```python
from build123d import *

# Parameters (mm, degrees)
SKETCH1_W                                 = 66.38
SKETCH1_H                                 = 120
BOSS_EXTRUDE1_DEPTH                       = 6.35
SKETCH2_W                                 = 40.98
SKETCH2_H                                 = 7.7
CUT_EXTRUDE1_DEPTH                        = 121
F_3_32_0_09375_DIAMETER_HOLE1_D           = 2.38125
F_3_32_0_09375_DIAMETER_HOLE1_DEPTH       = 19.05
F_3_32_0_09375_DIAMETER_HOLE1_CSINK_D     = 3.175
F_3_32_0_09375_DIAMETER_HOLE1_CSINK_ANGLE = 90
F_3_32_0_09375_DIAMETER_HOLE1_TIP         = 0.715399675
CUT_EXTRUDE2_DEPTH                        = 1
CUT_EXTRUDE2_DEPTH_BACK                   = 121
F_5_16_18_TAPPED_HOLE1_D                  = 6.5278
F_5_16_18_TAPPED_HOLE1_DEPTH              = 32.45
F_5_16_18_TAPPED_HOLE1_CSINK_D            = 9.2075
F_5_16_18_TAPPED_HOLE1_CSINK_ANGLE        = 90
F_5_16_18_TAPPED_HOLE1_TIP                = 1.961148974
CHAMFER1_SIZE                             = 3.175
SKETCH6_W                                 = 15.1
SKETCH6_H                                 = 7.75
CUT_EXTRUDE3_DEPTH                        = 6
FILLET1_R                                 = 1
SKETCH18_W                                = 14.39
SKETCH18_H                                = 120
CUT_EXTRUDE10_DEPTH                       = 13.7000001
SKETCH19_W                                = 5
SKETCH19_H                                = 12.7
BOSS_EXTRUDE3_DEPTH                       = 7.7
SKETCH20_W                                = 12.7
SKETCH20_H                                = 3
BOSS_EXTRUDE4_DEPTH                       = 1.1
CHAMFER3_SIZE                             = 1
CHAMFER4_SIZE                             = 2
SKETCH21_W                                = 12.7
SKETCH21_H                                = 100.95
CUT_EXTRUDE11_DEPTH                       = 7.7
SKETCH22_W                                = 24.87086649
SKETCH22_H                                = 0.4
CUT_EXTRUDE12_DEPTH                       = 121.0000001
SKETCH23_W                                = 40.98
SKETCH23_H                                = 0.68791644
CUT_EXTRUDE13_DEPTH                       = 121
CHAMFER5_SIZE                             = 2


with BuildPart() as part:
    # Sketch1 → Boss-Extrude1 (new body, symmetric)
    with BuildSketch(Plane(origin=(0, 0, 0), x_dir=(1, 0, 0), z_dir=(0, 1, 0))):
        with Locations((0, 60)):
            Rectangle(SKETCH1_W, SKETCH1_H)
    extrude(amount=BOSS_EXTRUDE1_DEPTH, both=True)

    # Sketch2 → Cut-Extrude1 (cut, through all)
    with BuildSketch(Plane.XY):
        with Locations((0, 2.5)):
            Rectangle(SKETCH2_W, SKETCH2_H)
    extrude(amount=-CUT_EXTRUDE1_DEPTH, mode=Mode.SUBTRACT)

    # 3_32 _0.09375_ Diameter Hole1
    with Locations(Plane.XY):
        with Locations((0, -3.35)):
            CounterSinkHole(F_3_32_0_09375_DIAMETER_HOLE1_D / 2, F_3_32_0_09375_DIAMETER_HOLE1_CSINK_D / 2, depth=F_3_32_0_09375_DIAMETER_HOLE1_DEPTH, counter_sink_angle=F_3_32_0_09375_DIAMETER_HOLE1_CSINK_ANGLE)
            with Locations((0, 0, -(F_3_32_0_09375_DIAMETER_HOLE1_DEPTH + F_3_32_0_09375_DIAMETER_HOLE1_TIP / 2))):  # 118° drill point
                Cone(0, F_3_32_0_09375_DIAMETER_HOLE1_D / 2, F_3_32_0_09375_DIAMETER_HOLE1_TIP, mode=Mode.SUBTRACT)

    # Sketch3 → Cut-Extrude2 (cut, two sides)
    with BuildSketch(Plane.XY) as cut_extrude2_sk:
        with BuildLine():
            Line((-140.137251951, -19.091259006), (-20.49, -6.35))
            ThreePointArc((-20.49, -6.35), (0, -5.26208356), (20.49, -6.35))
            Line((20.49, -6.35), (140.137251951, -19.091259006))
            Line((140.137251951, -19.091259006), (140.137251951, -259.738757065))
            Line((140.137251951, -259.738757065), (-140.137251951, -259.738757065))
            Line((-140.137251951, -259.738757065), (-140.137251951, -19.091259006))
        make_face()
    extrude(amount=CUT_EXTRUDE2_DEPTH, mode=Mode.SUBTRACT)
    extrude(cut_extrude2_sk.sketch, amount=-CUT_EXTRUDE2_DEPTH_BACK, mode=Mode.SUBTRACT)

    # 5_16-18 Tapped Hole1
    with Locations(Plane.XY):
        with Locations((-26.84, 0)):
            CounterSinkHole(F_5_16_18_TAPPED_HOLE1_D / 2, F_5_16_18_TAPPED_HOLE1_CSINK_D / 2, depth=F_5_16_18_TAPPED_HOLE1_DEPTH, counter_sink_angle=F_5_16_18_TAPPED_HOLE1_CSINK_ANGLE)
            with Locations((0, 0, -(F_5_16_18_TAPPED_HOLE1_DEPTH + F_5_16_18_TAPPED_HOLE1_TIP / 2))):  # 118° drill point
                Cone(0, F_5_16_18_TAPPED_HOLE1_D / 2, F_5_16_18_TAPPED_HOLE1_TIP, mode=Mode.SUBTRACT)

    # Chamfer1
    chamfer1_edges = [part.edges().sort_by_distance(p)[0] for p in [
        (-20.49, 6.35, -60),
    ]]
    chamfer(chamfer1_edges, length=CHAMFER1_SIZE)

    # Sketch6 → Cut-Extrude3 (cut, through all)
    with BuildSketch(Plane(origin=(0, -1.35, 0), x_dir=(1, 0, 0), z_dir=(0, 1, 0))):
        with Locations((3.55, 107.9216)):
            Rectangle(SKETCH6_W, SKETCH6_H)
        with Locations((-2.75, 47.6216)):
            Rectangle(SKETCH6_W, SKETCH6_H)
    extrude(amount=-CUT_EXTRUDE3_DEPTH, mode=Mode.SUBTRACT)

    # Fillet1
    fillet1_edges = [part.edges().sort_by_distance(p)[0] for p in [
        (11.1, -3.465359, -111.7966),
        (11.1, -3.465359, -104.0466),
        (-4, -3.326715824, -104.0466),
        (-4, -3.326715824, -111.7966),
        (4.8, -3.335813803, -51.4966),
        (4.8, -3.335813803, -43.7466),
        (-10.3, -3.443206194, -43.7466),
        (-10.3, -3.443206194, -51.4966),
    ]]
    fillet(fillet1_edges, radius=FILLET1_R)

    # Sketch18 → Cut-Extrude10 (cut, through all)
    with BuildSketch(Plane(origin=(0, 6.35, 0), x_dir=(1, 0, 0), z_dir=(0, 1, 0))):
        with Locations((25.995, 60)):
            Rectangle(SKETCH18_W, SKETCH18_H)
    extrude(amount=-CUT_EXTRUDE10_DEPTH, mode=Mode.SUBTRACT)

    # Sketch19 → Boss-Extrude3 (add)
    with BuildSketch(Plane(origin=(0, -1.35, 0), x_dir=(1, 0, 0), z_dir=(0, 1, 0))):
        with Locations((16.3, 19.05)):
            Rectangle(SKETCH19_W, SKETCH19_H)
        with Locations((16.3, 82.55)):
            Rectangle(SKETCH19_W, SKETCH19_H)
    extrude(amount=BOSS_EXTRUDE3_DEPTH)

    # Sketch20 → Boss-Extrude4 (add)
    with BuildSketch(Plane(origin=(18.8, 0, 0), x_dir=(0, 0, -1), z_dir=(1, 0, 0))):
        with Locations((19.05, 4.85)):
            Rectangle(SKETCH20_W, SKETCH20_H)
        with Locations((82.55, 4.85)):
            Rectangle(SKETCH20_W, SKETCH20_H)
    extrude(amount=BOSS_EXTRUDE4_DEPTH)

    # Chamfer3
    chamfer3_edges = [part.edges().sort_by_distance(p)[0] for p in [
        (19.9, 3.35, -82.55),
        (19.9, 3.35, -19.05),
    ]]
    chamfer(chamfer3_edges, length=CHAMFER3_SIZE)

    # Chamfer4
    chamfer4_edges = [part.edges().sort_by_distance(p)[0] for p in [
        (13.8, 6.35, -19.05),
        (13.8, 6.35, -82.55),
    ]]
    chamfer(chamfer4_edges, length=CHAMFER4_SIZE)

    # Sketch21 → Cut-Extrude11 (cut)
    with BuildSketch(Plane(origin=(0, 6.35, 0), x_dir=(1, 0, 0), z_dir=(0, 1, 0))):
        with Locations((-26.84, 69.525)):
            Rectangle(SKETCH21_W, SKETCH21_H)
    extrude(amount=-CUT_EXTRUDE11_DEPTH, mode=Mode.SUBTRACT)

    # Sketch22 → Cut-Extrude12 (cut, through all)
    with BuildSketch(Plane.XY):
        with Locations((0, -5.46208356)):
            Rectangle(SKETCH22_W, SKETCH22_H)
    extrude(amount=-CUT_EXTRUDE12_DEPTH, mode=Mode.SUBTRACT)

    # Sketch23 → Cut-Extrude13 (cut, through all)
    with BuildSketch(Plane.XY):
        with Locations((0, -6.00604178)):
            Rectangle(SKETCH23_W, SKETCH23_H)
    extrude(amount=-CUT_EXTRUDE13_DEPTH, mode=Mode.SUBTRACT)

    # Chamfer5
    chamfer5_edges = [part.edges().sort_by_distance(p)[0] for p in [
        (-2.75, -1.35, -51.4966),
        (4.8, -1.35, -47.6216),
        (-2.75, -1.35, -43.7466),
        (-10.3, -1.35, -47.6216),
        (-3.707106781, -1.35, -104.339493219),
        (10.807106781, -1.35, -104.339493219),
        (10.807106781, -1.35, -111.503706781),
        (4.507106781, -1.35, -51.203706781),
        (4.507106781, -1.35, -44.039493219),
        (-10.007106781, -1.35, -44.039493219),
        (-10.007106781, -1.35, -51.203706781),
        (-3.707106781, -1.35, -111.503706781),
        (3.55, -1.35, -104.0466),
        (-4, -1.35, -107.9216),
        (11.1, -1.35, -107.9216),
        (3.55, -1.35, -111.7966),
    ]]
    chamfer(chamfer5_edges, length=CHAMFER5_SIZE)


solid = part.part
```
Geometry check sheet. Reference: the model listing, model coordinates, mm. A direction names the side the tool comes from. Coordinates: 2 decimals unless noted, no trailing zeros. Loops run counter-clockwise (first coordinate to the right, second up) from the corner with the lowest first, then second, coordinate; pieces in that order, holes last. Notation, with made-up numbers: (82.5, 34.25) - (111.5, 34.25) arc R33 cw to (111.5, 64.25) - close; hole circle Ø5 at (46, -17). An arc over 180 degrees is marked (long way). One line per item, written item: value. Start each with the question number.
(1) Cross-section at A-A on y = 0. Enter the section's corners in (x, z).
(2) Cross-section at C-C on z = -87. Enter the section's corners in (x, y), plus the area to 3 significant figures.
(3) Cross-section at B-B on z = -15. Enter the section's corners in (x, y) (3 decimals).
(4) Material ranges on line 1 (X direction, y = 0, z = -15.5); line 2 (Z direction, x = 17, y = 3.25); line 3 (X direction, y = -3.35, z = -15), recorded low to high. Write a range as [from, to].
(5) Mould release check, pull along Z, two halves, no side actions. Record for faces 6 (the flat face through (17, 2, -25.4)), 7 (the flat face through (-2.842, -2.364, -52.483)), 8 (the flat face through (-33.19, -3, -46)), 9 (the flat face through (-8, -3, -120)): released by +Z, released by -Z, zero draft, split by the parting line, or undercut.
(6) Tool access check on faces 1 (the flat face through (18, 6.35, -83)), 2 (the flat face through (16, -5.662, -59)), 3 (the flat face through (-2.658, -2.364, -42.761)), 4 (the flat face through (14.79, 5.34, -18.96)), 5 (the flat face through (19.9, 5, -82)). Record the directions out of +Z, -Z, +X, -X, +Y, -Y that give a thin tool (end or side, any length) a straight path to the whole face; none if there is none.
(7) Depth check by flat-ended pin: P1, Ø2, axis at y = 0, z = -12.5, coming from the +X side; P2, Ø2, axis at x = -0.5, y = -4.5, coming from the +Z side; P3, Ø1.8, axis at x = 18, y = 0.5, coming from the +Z side; P4, Ø1, axis at x = -11, z = -70.5, coming from the -Y side. Enter the tip coordinate at first touch or a pass-through.
Results below:
1. outline: (-33.19, -19.05) - (-30.1, -19.05) - (-30.1, -1.34) - (-31.44, 0) - (-33.19, 0) - close; (-23.58, -19.05) - (-20.49, -19.05) - (-20.49, 0) - (-22.24, 0) - (-23.58, -1.34) - close; (13.8, -88.9) - (18.8, -88.9) - (18.8, -76.2) - (13.8, -76.2) - close; (13.8, -25.4) - (18.8, -25.4) - (18.8, -12.7) - (13.8, -12.7) - close
2. outline: (-33.19, -6.35) - (-20.49, -6.35) - (-20.49, -5.66) - (-12.44, -5.66) - (-12.44, -5.26) - (12.44, -5.26) - (12.44, -5.66) - (18.8, -5.66) - (18.8, 3.35) - (18.9, 3.35) - (19.9, 4.35) - (19.9, 6.35) - (15.8, 6.35) - (13.8, 4.35) - (13.8, -1.35) - (-33.19, -1.35) - close
2. area: 262 mm2
3. outline: (-33.19, -6.35) - (-20.49, -6.35) - (-20.49, -5.662) - (-12.435, -5.662) - (-12.435, -5.262) - (12.435, -5.262) - (12.435, -5.662) - (18.8, -5.662) - (18.8, 3.35) - (18.9, 3.35) - (19.9, 4.35) - (19.9, 6.35) - (15.8, 6.35) - (13.8, 4.35) - (13.8, -1.35) - (-20.49, -1.35) - (-20.49, 3.175) - (-23.665, 6.35) - (-33.19, 6.35) - close; hole circle Ø6.528 at (-26.84, 0); hole circle Ø2.381 at (0, -3.35)
4. line 1: x = [-33.19, -30.1], [-23.58, -20.49], [13.8, 18.8]
4. line 2: z = [-88.9, -76.2], [-25.4, -12.7]
4. line 3: x = [-33.19, -1.19], [1.19, 18.8]
5. face 6: undercut
5. face 7: undercut
5. face 8: zero draft
5. face 9: released by -Z
6. face 1: +Z, -Z, +X, -X, +Y
6. face 2: +Z, -Z, +X, -Y
6. face 3: +Y
6. face 4: +Z, -Z, +Y
6. face 5: +Z, -Z, +X, +Y, -Y
7. P1: stops at x = 18.8
7. P2: stops at z = 0
7. P3: stops at z = -12.7
7. P4: stops at y = -5.26
